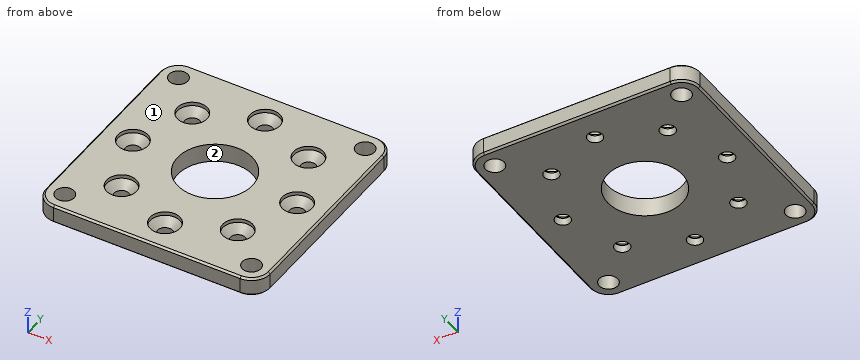
```python
from build123d import *

# Parameters (mm, degrees)
SKETCH_1_R          = 2.5
SKETCH_1_R_2        = 10
SKETCH_1_R_3        = 2
EXTRUDE_1_DEPTH     = 5
SKETCH_2_R          = 4
CUT_EXTRUDE_1_DEPTH = 1
CHAMFER_1_SIZE      = 2
CHAMFER1_SIZE       = 0.5


with BuildPart() as part:
    # 草图1 → 凸台-拉伸1 (new body)
    with BuildSketch(Plane.XY):
        with BuildLine():
            Line((-25, -30), (25, -30))
            ThreePointArc((25, -30), (28.535533906, -28.535533906), (30, -25))
            Line((30, -25), (30, 25))
            ThreePointArc((30, 25), (28.535533906, 28.535533906), (25, 30))
            Line((25, 30), (-25, 30))
            ThreePointArc((-25, 30), (-28.535533906, 28.535533906), (-30, 25))
            Line((-30, 25), (-30, -25))
            ThreePointArc((-30, -25), (-28.535533906, -28.535533906), (-25, -30))
        make_face()
        with Locations((-25, 25)):
            Circle(SKETCH_1_R, mode=Mode.SUBTRACT)
        with Locations(Location((-25, -25, 0), (0, 0, 180))):
            Circle(SKETCH_1_R, mode=Mode.SUBTRACT)
        with Locations((25, -25)):
            Circle(SKETCH_1_R, mode=Mode.SUBTRACT)
        with Locations(Location((25, 25, 0), (0, 0, 180))):
            Circle(SKETCH_1_R, mode=Mode.SUBTRACT)
        Circle(SKETCH_1_R_2, mode=Mode.SUBTRACT)
        with Locations((-15.556349186, 15.556349186)):
            Circle(SKETCH_1_R_3, mode=Mode.SUBTRACT)
        with Locations((0, 22)):
            Circle(SKETCH_1_R_3, mode=Mode.SUBTRACT)
        with Locations((15.556349186, 15.556349186)):
            Circle(SKETCH_1_R_3, mode=Mode.SUBTRACT)
        with Locations((22, 0)):
            Circle(SKETCH_1_R_3, mode=Mode.SUBTRACT)
        with Locations((15.556349186, -15.556349186)):
            Circle(SKETCH_1_R_3, mode=Mode.SUBTRACT)
        with Locations((0, -22)):
            Circle(SKETCH_1_R_3, mode=Mode.SUBTRACT)
        with Locations((-15.556349186, -15.556349186)):
            Circle(SKETCH_1_R_3, mode=Mode.SUBTRACT)
        with Locations((-22, 0)):
            Circle(SKETCH_1_R_3, mode=Mode.SUBTRACT)
    extrude(amount=EXTRUDE_1_DEPTH)

    # 草图2 → 切除-拉伸1 (cut)
    with BuildSketch(Plane.XY.offset(5)):
        with Locations((-15.556349186, 15.556349186)):
            Circle(SKETCH_2_R)
        with Locations((0, 22)):
            Circle(SKETCH_2_R)
        with Locations((15.556349186, 15.556349186)):
            Circle(SKETCH_2_R)
        with Locations((22, 0)):
            Circle(SKETCH_2_R)
        with Locations((15.556349186, -15.556349186)):
            Circle(SKETCH_2_R)
        with Locations((0, -22)):
            Circle(SKETCH_2_R)
        with Locations((-15.556349186, -15.556349186)):
            Circle(SKETCH_2_R)
        with Locations((-22, 0)):
            Circle(SKETCH_2_R)
    extrude(amount=-CUT_EXTRUDE_1_DEPTH, mode=Mode.SUBTRACT)

    # 倒角1
    chamfer_1_edges = [part.edges().sort_by_distance(p)[0] for p in [
        (13.556349186, -15.556349186, 4),
        (20, 0, 4),
        (13.556349186, 15.556349186, 4),
        (-2, 22, 4),
        (-17.556349186, 15.556349186, 4),
        (-24, 0, 4),
        (-17.556349186, -15.556349186, 4),
        (-2, -22, 4),
    ]]
    chamfer(chamfer_1_edges, length=CHAMFER_1_SIZE - 0.0001)  # a hair under: the kernel refuses the full size

    # Chamfer1
    chamfer1_edges = [part.edges().sort_by_distance(p)[0] for p in [
        (-30, 0, 0),
        (-28.535533906, 28.535533906, 0),
        (0, 30, 0),
        (28.535533906, 28.535533906, 0),
        (-28.535533906, 28.535533906, 5),
        (-30, 0, 5),
        (-28.535533906, -28.535533906, 5),
        (0, -30, 5),
        (28.535533906, -28.535533906, 5),
        (30, 0, 5),
        (28.535533906, 28.535533906, 5),
        (30, 0, 0),
        (0, 30, 5),
        (28.535533906, -28.535533906, 0),
        (0, -30, 0),
        (-28.535533906, -28.535533906, 0),
    ]]
    chamfer(chamfer1_edges, length=CHAMFER1_SIZE)


solid = part.part
```
Work out the finished part from the listing and answer in its coordinate system (mm). Face numbers are marked on the shaded views. Round coordinates to 2 decimals unless told otherwise and drop trailing zeros. Write each loop counter-clockwise with the first axis right and the second up, starting at its lowest first coordinate (ties: lowest second). Pieces come first, ordered by that corner, then holes. Notation, with made-up numbers: (77, -7.75) -> (134, -7.75) arc R21 cw to (134, 22.25) -> close; hole circle Ø7 at (67.25, 71). An arc over 180 degrees is marked (long way). Write each question's results on one line, items separated by ' | '.
1) The part is cut by section D-D (y = -7.5). Write down the section's boundary in (x, z).
Findings:
outline: (-30, 0.5) -> (-29.5, 0) -> (-6.61, 0) -> (-6.61, 5) -> (-29.5, 5) -> (-30, 4.5) -> close; (6.61, 0) -> (29.5, 0) -> (30, 0.5) -> (30, 4.5) -> (29.5, 5) -> (6.61, 5) -> close
2) The part is cut by section A-A (x = 0). State how many separate pieces and enclosed holes the cut face has, and give its area (3 significant figures).
Findings:
separate pieces: 4 | enclosed holes: 0 | area: 144 mm²
3) Flat-ended cylindrical pins translate along their axes: pin 1 (2.5 mm diameter, centred on x = -1, y = -23.5, fed in from +Z); pin 2 (3 mm diameter, centred on x = 22, y = 0, fed in from -Z); pin 3 (2 mm diameter, centred on x = 8, y = -15, fed in from -Z); pin 4 (1.5 mm diameter, centred on x = -17, y = -15, fed in from +Z). Find the tip coordinate at first contact, or state that the pin passes through.
Findings:
pin 1: stops at z = 3.05 | pin 2: passes through | pin 3: stops at z = 0 | pin 4: stops at z = 2.3
4) For a pull along X with two mould halves and no side action, classify the marked faces 1 and 2 as +X half, -X half, draft (parallel to the pull), parting line (faces both ways), or undercut.
Findings:
face 1: draft | face 2: undercut
5) Consider line 1 along Y through (x, z) = (-25, 1.75); line 2 along X through (y, z) = (15.5, 1.9); line 3 along X through (y, z) = (1, 4.05). Determine where each line is inside the solid, lowest interval first. Write a range as [from, to].
Findings:
line 1: y = [-30, -27.5], [-22.5, 22.5], [27.5, 30] | line 2: x = [-30, -17.56], [-13.56, 13.56], [17.56, 30] | line 3: x = [-30, -25.87], [-18.13, -9.95], [9.95, 18.13], [25.87, 30]
